Model file for the job. Use its own axes, mm. Round coordinates to 2 decimals unless told otherwise and drop trailing zeros. Write each loop counter-clockwise with the first axis right and the second up, starting at its lowest first coordinate (ties: lowest second). Pieces come first, ordered by that corner, then holes.
```python
from build123d import *

# Parameters (mm, degrees)
F0_R     = 6.35
F1_DEPTH = 57.15
F2_R     = 3.175
F3_DEPTH = 12.7
F5_D     = 5.5118
F5_DEPTH = 12.7
F5_TIP   = 1.65591178


with BuildPart() as f1:
    # F0 (on Front) → F1 (new body)
    with BuildSketch(Plane.XZ):
        Circle(F0_R)
    extrude(amount=F1_DEPTH)

    # F2 (on face) → F3 (join)
    with BuildSketch(Plane.XZ.offset(57.15)):
        Circle(F2_R)
    extrude(amount=F3_DEPTH)

    # F5
    with Locations(Plane(origin=(0, 0, 0), x_dir=(-1, 0, 0), z_dir=(0, 1, 0))):
        with Locations((0, 0)):
            Hole(F5_D / 2, depth=F5_DEPTH)
            with Locations((0, 0, -(F5_DEPTH + F5_TIP / 2))):  # 118° drill point
                Cone(0, F5_D / 2, F5_TIP, mode=Mode.SUBTRACT)


solid = f1.part
```
1) Cut at A-A on y = -4.5. List the corners of the cut face in (x, z), and give its area (3 significant figures).
2) Cut at D-D on z = -4.25. List the corners of the cut face in (x, y).
3) Cut at C-C on x = -5.25. List the corners of the cut face in (y, z).
4) Cut at B-B on y = -47. List the corners of the cut face in (x, z), and give its area (3 significant figures).
5) Wall check: probe 1 along Z at (x, y) = (0, -7); probe 2 along Y at (x, z) = (-4.75, -2.5); probe 3 along Z at (x, y) = (5, -31). Give the ranges that are in metal, low to high.
6) Flat gauge pins, fed straight in: pin 1 Ø3 at (x, y) = (3, -53) entering from +Z; pin 2 Ø3 at (x, z) = (-4.5, 5) entering from -Y; pin 3 Ø3 at (x, y) = (-2.5, -10.5) entering from +Z. Where does each tip first touch, or does it go through?
7) Pull direction X, two halves, no side cores. Call faces 1 (the face through (-0.6, -6.44, -2.69)), 2 (the face through (-0.69, -63.41, -3.1)), 3 (the face through (-2, -57.15, 3)): released by +X, released by -X, zero draft, split by the parting line, or undercut.
Result sheet:
1. outline: circle Ø12.7 at (0, 0); hole circle Ø5.51 at (0, 0)
1. area: 103 mm2
2. outline: (-4.72, -57.15) - (4.72, -57.15) - (4.72, 0) - (-4.72, 0) - close
3. outline: (-57.15, -3.57) - (0, -3.57) - (0, 3.57) - (-57.15, 3.57) - close
4. outline: circle Ø12.7 at (0, 0)
4. area: 127 mm2
5. probe 1: z = -6.35 to -2.76, 2.76 to 6.35
5. probe 2: y = -57.15 to 0
5. probe 3: z = -3.91 to 3.91
6. pin 1: stops at z = 6.17
6. pin 2: stops at y = -57.15
6. pin 3: stops at z = 6.27
7. face 1: undercut
7. face 2: split by the parting line
7. face 3: zero draft
